Could you check a few things on this model? Use its own coordinates, in mm. Face numbers are marked on the shaded views. Give positions to 0.01 mm unless a question says otherwise; leave off trailing zeros. Order: outer loops, then holes, each group sorted by start corner. A loop starts at its lowest first (then second) coordinate and runs counter-clockwise, first axis right, second up. Notation, with made-up numbers: M 43,-37 L 64,-37 A24 cw 64,-18 Z; hole C 3,38 d5. An arc over 180 degrees is marked long. Use a Markdown table: item, result. Add a question column.
```python
from build123d import *

# Parameters (mm, degrees)
F2_DEPTH = 2.5
F4_DEPTH = 2
F5_T     = -2


with BuildPart() as f2:
    # F1 (on Top) → F2 (new body)
    with BuildSketch(Plane.XY):
        with BuildLine():
            Line((23.5, 27.5), (-23.5, 27.5))
            ThreePointArc((-23.5, 27.5), (-26.3284271247, 26.3284271247), (-27.5, 23.5))
            Line((-27.5, 23.5), (-27.5, -23.5))
            ThreePointArc((-27.5, -23.5), (-26.3284271247, -26.3284271247), (-23.5, -27.5))
            Line((-23.5, -27.5), (23.5, -27.5))
            ThreePointArc((23.5, -27.5), (26.3284271247, -26.3284271247), (27.5, -23.5))
            Line((27.5, -23.5), (27.5, 23.5))
            ThreePointArc((27.5, 23.5), (26.3284271247, 26.3284271247), (23.5, 27.5))
        make_face()
    extrude(amount=F2_DEPTH)

    # F3 (on face) → F4 (join)
    with BuildSketch(Plane.XY.offset(2.5)):
        with BuildLine():
            Line((21, 25), (-21, 25))
            ThreePointArc((-21, 25), (-23.8284271247, 23.8284271247), (-25, 21))
            Line((-25, 21), (-25, -21))
            ThreePointArc((-25, -21), (-23.8284271247, -23.8284271247), (-21, -25))
            Line((-21, -25), (21, -25))
            ThreePointArc((21, -25), (23.8284271247, -23.8284271247), (25, -21))
            Line((25, -21), (25, 21))
            ThreePointArc((25, 21), (23.8284271247, 23.8284271247), (21, 25))
        make_face()
    extrude(amount=F4_DEPTH)

    # F5
    f5_openings = [f2.faces().sort_by_distance(p)[0] for p in [
        (0, 0, 4.5),
    ]]
    offset(amount=F5_T, openings=f5_openings, kind=Kind.INTERSECTION)


solid = f2.part
```
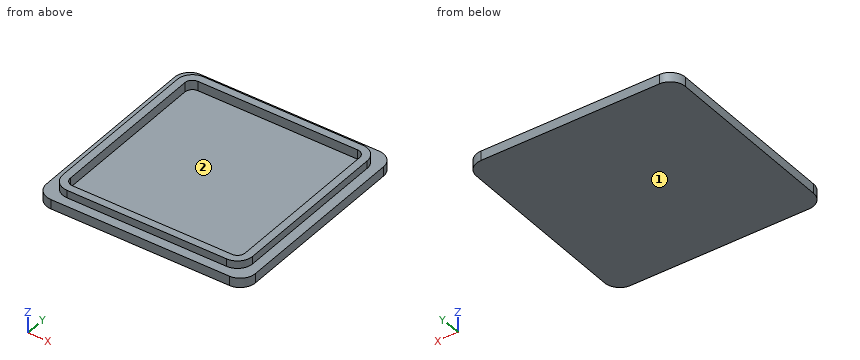
1) For pin 1 (1.6 mm diameter, centred on x = 7.5, z = 4, fed in from -Y); pin 2 (1.6 mm diameter, centred on x = -0.5, z = 3.5, fed in from +Y); pin 3 (1.2 mm diameter, centred on y = -5.5, z = 3.5, fed in from -X); pin 4 (1.6 mm diameter, centred on y = -5.5, z = 3, fed in from +X), each with a flat end and sliding along its axis, tell me the tip position at first contact or that it passes through.
2) Suppose I cut it at B-B on z = 3.65. Please give me the cut outline in (x, y), and give its area (3 significant figures).
3) Please list where these lines run through material, in increasing order: line 1 (X direction, y = 4, z = 3.1); line 2 (X direction, y = -15, z = 2.15). Write a range as from..to.
4) Suppose I cut it at A-A on x = 5.5. Please give me the cut outline in (y, z), and give its area (4 significant figures).
5) We'd pull the mould along Y, two halves only. Please class the marked faces 1 and 2: pulls with the +Y half, pulls with the -Y half, needs draft (parallel to the pull), parting line crosses it, or undercut.
Values found:
| question | item | result |
|---|---|---|
| 1 | pin 1 | stops at y = -25 |
| 1 | pin 2 | stops at y = 25 |
| 1 | pin 3 | stops at x = -25 |
| 1 | pin 4 | stops at x = 27.5 |
| 2 | outline | M -25,-21 A4 ccw -21,-25 L 21,-25 A4 ccw 25,-21 L 25,21 A4 ccw 21,25 L -21,25 A4 ccw -25,21 Z; hole M -23,-21 A2 ccw -21,-23 L 21,-23 A2 ccw 23,-21 L 23,21 A2 ccw 21,23 L -21,23 A2 ccw -23,21 Z |
| 2 | area | 374 mm^2 |
| 3 | line 1 | x = -25..-23, 23..25 |
| 3 | line 2 | x = -27.5..-23, 23..27.5 |
| 4 | outline | M -27.5,0 L 27.5,0 L 27.5,2.5 L 25,2.5 L 25,4.5 L 23,4.5 L 23,2 L -23,2 L -23,4.5 L -25,4.5 L -25,2.5 L -27.5,2.5 Z |
| 4 | area | 122.5 mm^2 |
| 5 | face 1 | needs draft |
| 5 | face 2 | undercut |
